Geometry check sheet. Reference: the model listing, model coordinates, mm. Face numbers are marked on the shaded views. A direction names the side the tool comes from. Round coordinates to 2 decimals unless told otherwise and drop trailing zeros. Order: outer loops, then holes, each group sorted by start corner. A loop starts at its lowest first (then second) coordinate and runs counter-clockwise, first axis right, second up.
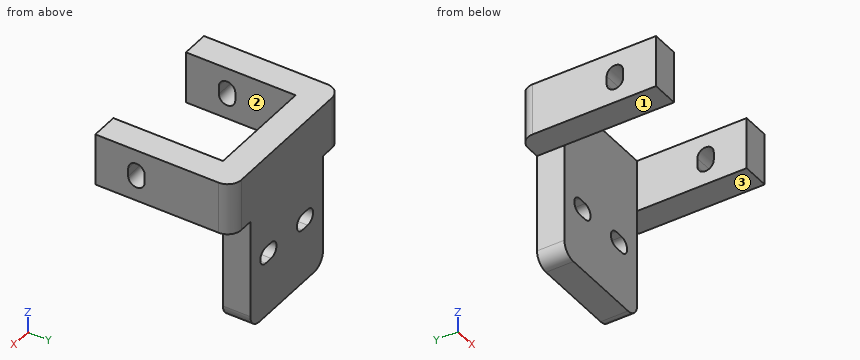
Autodesk Inventor part; units mm, degrees
ref_plane "YZ Plane" through (0, 0, 0) normal (1, 0, 0) x (0, 1, 0)
ref_plane "XZ Plane" through (0, 0, 0) normal (0, 1, 0) x (-1, 0, 0)
ref_plane "XY Plane" through (0, 0, 0) normal (0, 0, 1) x (1, 0, 0)
sketch "Sketch1" plane through (0, 0, 0) normal (0, 0, 1) x (1, 0, 0)
  line L0 (-20.15, 20) -> (20.15, 20)
  line L1 (20.15, 20) -> (20.15, -20)
  line L2 (20.15, -20) -> (-20.15, -20)
  line L3 (-20.15, -20) -> (-20.15, 20)
  line L4 (30.15, 30) -> (-30.15, 30)
  line L5 (-30.15, 30) -> (-30.15, -30)
  line L6 (-30.15, -30) -> (30.15, -30)
  line L7 (30.15, -30) -> (30.15, 30)
  line L8 (-20.15, -20) -> (-30.15, -20)
  line L9 (20.15, -20) -> (30.15, -20)
  point P0 (0, 0)
  point P1 (0, 20)
  point P2 (-20.15, 0)
  dimension "d0" = 40.3
  dimension "d1" = 40
  dimension "d2" = 10
extrude "Extrusion1" add sketch "Sketch1" along normal blind 60 contours L3 L8 L5 L4 L7 L9 L1 L0
sketch "Sketch3" plane through (30.15, -20, 0) normal (1, 0, 0) x (0, 0, -1)
  line L0 (-41, 40) -> (0, 40)
  line L1 (0, 40) -> (0, 0)
  line L2 (0, 0) -> (-41, 0)
  line L3 (-41, 0) -> (-41, 40)
  line L4 (-60, 0) -> (-60, 50)
  line L5 (0, 0) -> (-60, 0)
  line L6 (0, 50) -> (-60, 50)
  line L7 (0, 0) -> (0, 50)
  point P0 (0, 20)
  dimension "d5" = 19
  dimension "d6" = 10
extrude "Extrusion2" cut sketch "Sketch3" against normal through all contours L0 L1 L2 L3
sketch "Sketch5" plane through (-30.15, 20, 0) normal (0, -1, 0) x (1, 0, 0)
  line L0 (60.3, 41) -> (50.3, 41)
  line L1 (50.3, 41) -> (50.3, 0)
  line L2 (50.3, 0) -> (60.3, 0)
  line L3 (60.3, 0) -> (60.3, 41)
  line L4 (60.3, 41) -> (60.3, 0)
  line L5 (0, 0) -> (60.3, 0)
  line L6 (60.3, 41) -> (50.3, 41)
  line L7 (50.3, 41) -> (50.3, 60)
  point P0 (30.15, 0)
extrude "Extrusion4" cut sketch "Sketch5" against normal through all
mirror "Mirror1" about plane through (0, 0, 0) normal (1, 0, 0) of "Extrusion4"
fillet "Fillet1" radius 5 4 edges at (-30.15, 30, 50.5) (30.15, 30, 50.5) (-20.15, 25, 0) (20.15, 25, 0)
sketch "Sketch9" plane through (30.15, -20, 60) normal (1, 0, 0) x (0, 0, -1)
  line L0 (8, 15) -> (11, 15) construction
  line L1 (8, 12) -> (11, 12)
  line L2 (11, 18) -> (8, 18)
  arc A0 (8, 18) -> (8, 12) centre (8, 15) ccw
  arc A1 (11, 12) -> (11, 18) centre (11, 15) ccw
  line L3 (19, 0) -> (0, 0)
  point P0 (60, 20)
  point P1 (9.5, 15)
  point P2 (9.5, 0)
  dimension "d34" = 3
  dimension "d35" = 6
  dimension "d36" = 15
extrude "Extrusion5" cut sketch "Sketch9" against normal through all
sketch "Sketch10" plane through (-15.15, 30, 0) normal (0, 1, 0) x (1, 0, 0)
  line L0 (3.5, -23) -> (6.5, -23) construction
  line L1 (3.5, -26) -> (6.5, -26)
  line L2 (6.5, -20) -> (3.5, -20)
  arc A0 (3.5, -20) -> (3.5, -26) centre (3.5, -23) ccw
  arc A1 (6.5, -26) -> (6.5, -20) centre (6.5, -23) ccw
  line L3 (23.8, -23) -> (26.8, -23) construction
  line L4 (23.8, -26) -> (26.8, -26)
  line L5 (26.8, -20) -> (23.8, -20)
  arc A2 (23.8, -20) -> (23.8, -26) centre (23.8, -23) ccw
  arc A3 (26.8, -26) -> (26.8, -20) centre (26.8, -23) ccw
  line L6 (-5, -5) -> (-5, -41)
  line L7 (35.3, -41) -> (35.3, -5)
  point P0 (15.15, 0)
  point P1 (5, -23)
  point P2 (25.3, -23)
  point P3 (-5, -23)
  dimension "d39" = 3
  dimension "d40" = 6
  dimension "d41" = 10
  dimension "d42" = 10
extrude "Extrusion6" cut sketch "Sketch10" against normal through all
properties part number "0008-10-032 Suport cadru si axa Z" material "ABS Plastic"
(1) Set-up check for the marked faces 1, 2 and 3: record each of +Z, -Z, +X, -X, +Y, -Y from which the full face is reachable in a straight line by a thin tool's end or side.
Returned:
face 1: -Z, -X, +Y, -Y
face 2: +Z, -Z, -Y
face 3: -Z, +X, +Y, -Y
(2) Sectioned sample at D-D, the plane x = -21. Record the cut outline in (y, z), and give its area (3 significant figures).
Returned:
outline: (-20, 41) - (30, 41) - (30, 60) - (-20, 60) - close; hole (-8, 49) arc R3 ccw to (-2, 49) - (-2, 52) arc R3 ccw to (-8, 52) - close
area: 904 mm2
(3) Sectioned sample at A-A, the plane y = 16. Record the cut outline in (x, z), and give its area (3 significant figures).
Returned:
outline: (-30.15, 41) - (-20.15, 41) - (-20.15, 60) - (-30.15, 60) - close; (20.15, 41) - (30.15, 41) - (30.15, 60) - (20.15, 60) - close
area: 380 mm2
(4) Sectioned sample at C-C, the plane x = 10. Record the cut outline in (y, z), and give its area (3 significant figures).
Returned:
outline: (20, 0) - (30, 0) - (30, 20) - (20, 20) - close; (20, 26) - (30, 26) - (30, 60) - (20, 60) - close
area: 540 mm2
(5) Sectioned sample at B-B, the plane z = 23. Record the cut outline in (x, y), and give its area (3 significant figures).
Returned:
outline: (-20.15, 20) - (-14.65, 20) - (-14.65, 30) - (-20.15, 30) - close; (-5.65, 20) - (5.65, 20) - (5.65, 30) - (-5.65, 30) - close; (14.65, 20) - (20.15, 20) - (20.15, 30) - (14.65, 30) - close
area: 223 mm2
(6) Depth check by flat-ended pin: P1, Ø11, axis at y = 24, z = 14.5, coming from the -X side; P2, Ø5, axis at y = 26.5, z = 26.5, coming from the +X side; P3, Ø3, axis at x = -15.5, z = 53, coming from the -Y side. Enter the tip coordinate at first touch or a pass-through.
Returned:
P1: stops at x = -20.15
P2: stops at x = 20.15
P3: stops at y = 20
(7) Material ranges on line 1 (X direction, y = 2.5, z = 48.5); line 2 (Z direction, x = -20.5, y = 2); line 3 (Y direction, x = -13.5, z = 41), recorded low to high.
Returned:
line 1: x = -30.15 to -20.15, 20.15 to 30.15
line 2: z = 41 to 60
line 3: y = 20 to 30
